Can you work these out from the model? Positions are in its coordinate system, mm. Round coordinates to 2 decimals unless told otherwise and drop trailing zeros. Loops run counter-clockwise (first coordinate to the right, second up) from the corner with the lowest first, then second, coordinate; pieces in that order, holes last.
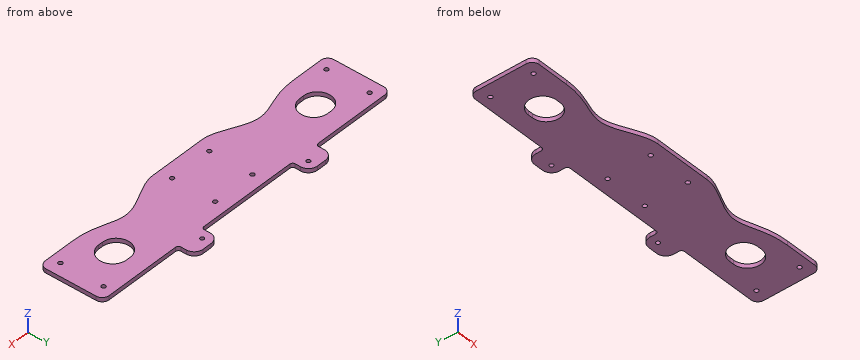
```python
from build123d import *

# Parameters (mm, degrees)
SKETCH1_W           = 119.75
SKETCH1_H           = 50
BOSS_EXTRUDE1_DEPTH = 3
SKETCH2_R           = 1.5
CUT_EXTRUDE1_DEPTH  = 3
SKETCH3_R           = 1.4
BOSS_EXTRUDE2_DEPTH = 3
FILLET1_R           = 2
CUT_EXTRUDE2_DEPTH  = 10
FILLET2_R           = 5
CUT_EXTRUDE3_DEPTH  = 10


with BuildPart() as part:
    # Sketch1 → Boss-Extrude1 (new body)
    with BuildSketch(Plane.XY):
        with Locations((59.875, 25)):
            Rectangle(SKETCH1_W, SKETCH1_H)
    extrude(amount=BOSS_EXTRUDE1_DEPTH)

    # Sketch2 → Cut-Extrude1 (cut)
    with BuildSketch(Plane(origin=(0, 0, 0), x_dir=(-1, 0, 0), z_dir=(0, 0, -1))):
        with Locations((-104.25, 40.5)):
            Circle(SKETCH2_R)
        with Locations((-104.25, 9.5)):
            Circle(SKETCH2_R)
        with Locations((-9, 42.5)):
            Circle(SKETCH2_R)
        with Locations((-9, 11.5)):
            Circle(SKETCH2_R)
    extrude(amount=-CUT_EXTRUDE1_DEPTH, mode=Mode.SUBTRACT)

    # Mirror1: part across plane


with BuildPart() as part_1:
    add(part.part)
    add(part.part.mirror(Plane(origin=(119.75, 0, 3), x_dir=(0, 0, 1), z_dir=(-1, 0, 0))))

    # Sketch3 → Boss-Extrude2 (add)
    with BuildSketch(Plane(origin=(0, 0, 0), x_dir=(-1, 0, 0), z_dir=(0, 0, -1))):
        with BuildLine():
            Line((-82, 50), (-82, 56))
            ThreePointArc((-82, 56), (-80.096194078, 60.596194078), (-75.5, 62.5))
            Line((-75.5, 62.5), (-68.843823796, 62.5))
            ThreePointArc((-68.843823796, 62.5), (-64.247629718, 60.596194078), (-62.343823796, 56))
            Line((-62.343823796, 56), (-62.343823796, 50))
            Line((-62.343823796, 50), (-82, 50))
        make_face()
        with Locations((-75.5, 56)):
            Circle(SKETCH3_R, mode=Mode.SUBTRACT)
    boss_extrude2 = extrude(amount=-BOSS_EXTRUDE2_DEPTH)

    # Mirror2: Boss-Extrude2 across plane
    add(boss_extrude2.mirror(Plane(origin=(119.75, 0, 0), x_dir=(0, 0, 1), z_dir=(1, 0, 0))))

    # Fillet1
    fillet1_edges = [part_1.edges().sort_by_distance(p)[0] for p in [
        (177.156176204, 50, 1.5),
        (157.5, 50, 1.5),
        (62.343823796, 50, 1.5),
        (82, 50, 1.5),
    ]]
    fillet(fillet1_edges, radius=FILLET1_R)

    # Sketch4 → Cut-Extrude2 (cut)
    with BuildSketch(Plane(origin=(0, 0, 0), x_dir=(-1, 0, 0), z_dir=(0, 0, -1))):
        with BuildLine():
            Line((-27.655095692, 4), (0, 4))
            Line((0, 4), (0, 0))
            Line((0, 0), (-99.256160352, 0))
            add(Edge.make_bspline(
                [(-99.256160352, 0), (-90.116604623, 0), (-79.005268065, 8.449150394), (-62.736804921, 12.15262313), (-50.625142782, 8.672513345), (-38.701859446, 4), (-27.655095692, 4)],
                knots=[0, 0, 0, 0, 0.434613944, 0.535270934, 0.727022104, 1, 1, 1, 1], degree=3))
        make_face()
    cut_extrude2 = extrude(amount=-CUT_EXTRUDE2_DEPTH, mode=Mode.SUBTRACT)

    # Mirror3: Cut-Extrude2 across plane
    add(cut_extrude2.mirror(Plane(origin=(119.75, 0, 0), x_dir=(0, 0, 1), z_dir=(1, 0, 0))), mode=Mode.SUBTRACT)

    # Fillet2
    fillet2_edges = [part_1.edges().sort_by_distance(p)[0] for p in [
        (239.5, 4, 1.5),
        (239.5, 50, 1.5),
        (0, 4, 1.5),
        (0, 50, 1.5),
    ]]
    fillet(fillet2_edges, radius=FILLET2_R)

    # Sketch5 → Cut-Extrude3 (cut)
    with BuildSketch(Plane(origin=(0, 0, 0), x_dir=(-1, 0, 0), z_dir=(0, 0, -1))):
        with BuildLine():
            Line((-34.5, 17), (-37.5, 17))
            ThreePointArc((-37.5, 17), (-47.5, 27), (-37.5, 37))
            Line((-37.5, 37), (-34.5, 37))
            ThreePointArc((-34.5, 37), (-24.5, 27), (-34.5, 17))
        make_face()
    cut_extrude3 = extrude(amount=-CUT_EXTRUDE3_DEPTH, mode=Mode.SUBTRACT)

    # Mirror4: Cut-Extrude3 across plane
    add(cut_extrude3.mirror(Plane(origin=(119.75, 0, 0), x_dir=(0, 0, 1), z_dir=(1, 0, 0))), mode=Mode.SUBTRACT)


solid = part_1.part
```
(1) Suppose I cut it at B-B (x = 110.5). Write out the boundary of the cut face in (y, z), then the cut area to 3 significant figures.
(2) For pin 1 (2.5 mm diameter, centred on x = 9, y = 11.5, fed in from -Z); pin 2 (0.9 mm diameter, centred on x = 203.5, z = 2, fed in from -Y); pin 3 (0.9 mm diameter, centred on x = 107, z = 1.5, fed in from +Y), each with a flat end and sliding along its axis, tell me the tip position at first contact or that it passes through.
(3) If I drill on line 1 (Y direction, x = 104.25, z = 1.7); line 2 (X direction, y = 43, z = 1.05); line 3 (Y direction, x = 103, z = 2.15), over which ranges is the centre line in solid material (lowest first)?
(4) Suppose I cut it at A-A (z = 1.65). Give the number of separate pieces and of enclosed holes in the cut face, then the cut area to 3 significant figures.
Check result:
1. outline: (0, 0) - (50, 0) - (50, 3) - (0, 3) - close
1. area: 150 mm2
2. pin 1: passes through
2. pin 2: stops at y = 4.5
2. pin 3: stops at y = 50
3. line 1: y = 0 to 8, 11 to 39, 42 to 50
3. line 2: x = 0 to 7.59, 10.41 to 229.09, 231.91 to 239.5
3. line 3: y = 0 to 8.67, 10.33 to 39.67, 41.33 to 50
4. separate pieces: 1
4. enclosed holes: 12
4. area: 10,400 mm2
